The listing builds one solid part. Answer for the finished solid, in the listing's coordinates (mm). A direction names the side the tool comes from. Round coordinates to 2 decimals unless told otherwise and drop trailing zeros. Write each loop counter-clockwise with the first axis right and the second up, starting at its lowest first coordinate (ties: lowest second). Pieces come first, ordered by that corner, then holes. Notation, with made-up numbers: M 21,83 L 37,83 A17 ccw 37,116 Z; hole C -36.5,15 d2. An arc over 180 degrees is marked long. One line per item, written item: value. Start each with the question number.
(1) Consider probe 1 along Y at (x, z) = (2, 0.5); probe 2 along X at (y, z) = (1.2, 0); probe 3 along X at (y, z) = (-52, -0.75). Determine where each line is inside the solid, lowest interval first.
(2) For a pull along Z with two mould halves and no side action, classify faces 6 (the cylindrical face through (-4.21, 0.99, -0.38)), 7 (the cylindrical face through (4.285, -53.986, 4.199)), 8 (the flat face through (0, -53, 0)) as released by +Z, released by -Z, zero draft, split by the parting line, or undercut.
(3) Section C-C (x = 1.25) is taken. Determine the outline of the cut face in (y, z), plus the area to 3 significant figures.
(4) Given P1, Ø1.5, axis at x = 3, z = 2, coming from the +Y side; P2, Ø0.6, axis at y = 3, z = 0.5, coming from the -X side; P3, Ø4.5, axis at x = -2.5, z = 0, coming from the -Y side, each flat-ended and moving along its own axis, determine where each tip first touches the part or whether it passes through.
(5) For faces 1 (the flat face through (4, 3, -1)), 2 (the flat face through (-2, 0, -2)), 3 (the cylindrical face through (4.285, 2.986, 4.199)), 4 (the flat face through (4, -54, -1)), 5 (the flat face through (5, 4, 0)), determine the directions among +Z, -Z, +X, -X, +Y, -Y from which every point of the face is accessible in a straight line to the end or side of a thin tool.
(6) Section A-A (z = 0) is taken. Determine the outline of the cut face in (x, y).
(7) Section B-B (x = -2.5) is taken. Determine the outline of the cut face in (y, z), plus the area to 3 significant figures.
(8) Section D-D (z = 2.25) is taken. Determine the outline of the cut face in (x, y), plus the area to 3 significant figures.
```python
from build123d import *

# Parameters (mm, degrees)
SKETCH1_R           = 1.75
BOSS_EXTRUDE3_DEPTH = 2
BOSS_EXTRUDE4_DEPTH = 25.5
BOSS_EXTRUDE5_DEPTH = 4


with BuildPart() as part:
    # Sketch1 → Boss-Extrude3 (new body)
    # profile 1 of 3: a face of its own
    with BuildSketch(Plane(origin=(0, 0, 0), x_dir=(1, 0, 0), z_dir=(0, 1, 0))):
        with BuildLine():
            Line((0.004495957, 4.5), (-3.991008085, 4.5))
            ThreePointArc((-3.991008085, 4.5), (-7.240580672, 0), (-3.991008085, -4.5))
            Line((-3.991008085, -4.5), (0.004495957, -4.5))
            ThreePointArc((0.004495957, -4.5), (2.65, 0), (0.004495957, 4.5))
        make_face()
        with Locations(Location((-2.5, 0, 0), (0, 0, 270))):
            Circle(SKETCH1_R, mode=Mode.SUBTRACT)
    # profile 2 of 3: a face of its own
    with BuildSketch(Plane(origin=(0, 0, 0), x_dir=(1, 0, 0), z_dir=(0, 1, 0))):
        with BuildLine():
            Line((4, 4.5), (0.004495957, 4.5))
            ThreePointArc((0.004495957, 4.5), (2.65, 0), (0.004495957, -4.5))
            Line((0.004495957, -4.5), (4, -4.5))
            Line((4, -4.5), (5, -4.5))
            ThreePointArc((5, -4.5), (4.292893219, -4.207106781), (4, -3.5))
            Line((4, -3.5), (4, 4.5))
        make_face()
    # profile 3 of 3: a face of its own
    with BuildSketch(Plane(origin=(0, 0, 0), x_dir=(1, 0, 0), z_dir=(0, 1, 0))):
        with BuildLine():
            Line((5.019474666, 4.5), (4, 4.5))
            Line((4, 4.5), (4, -3.5))
            ThreePointArc((4, -3.5), (4.292893219, -4.207106781), (5, -4.5))
            Line((5, -4.5), (7, -4.5))
            Line((7, -4.5), (7, 4.5))
            Line((7, 4.5), (5.019474666, 4.5))
        make_face()
    extrude(amount=BOSS_EXTRUDE3_DEPTH)

    # Sketch1_3 → Boss-Extrude4 (add)
    with BuildSketch(Plane(origin=(0, 0, 0), x_dir=(1, 0, 0), z_dir=(0, 1, 0))):
        with BuildLine():
            ThreePointArc((0.004495957, 4.5), (2.65, 0), (0.004495957, -4.5))
            Line((0.004495957, -4.5), (7, -4.5))
            Line((7, -4.5), (7, 4.5))
            Line((7, 4.5), (0.004495957, 4.5))
        make_face()
    extrude(amount=-BOSS_EXTRUDE4_DEPTH)

    # Sketch1_5 → Boss-Extrude5 (add)
    with BuildSketch(Plane(origin=(0, 0, 0), x_dir=(1, 0, 0), z_dir=(0, 1, 0))):
        with BuildLine():
            Line((5.019474666, 4.5), (4, 4.5))
            Line((4, 4.5), (4, -3.5))
            ThreePointArc((4, -3.5), (4.292893219, -4.207106781), (5, -4.5))
            Line((5, -4.5), (7, -4.5))
            Line((7, -4.5), (7, 4.5))
            Line((7, 4.5), (5.019474666, 4.5))
        make_face()
    extrude(amount=BOSS_EXTRUDE5_DEPTH)

    # Mirror1: part across plane


with BuildPart() as part_1:
    add(part.part)
    add(part.part.mirror(Plane.ZX.offset(-25.5)))


solid = part_1.part
```
Recorded:
1. probe 1: y = -53 to -51, 0 to 2
1. probe 2: x = -7.24 to -4.25, -0.75 to 7
1. probe 3: x = -7.18 to -4.08, -0.92 to 7
2. face 6: undercut
2. face 7: released by +Z
2. face 8: zero draft
3. outline: M -53,-4.5 L 2,-4.5 L 2,4.5 L -53,4.5 Z; hole M -51,-3.53 L 0,-3.53 L 0,3.53 L -51,3.53 Z
3. area: 135 mm2
4. P1: stops at y = 2
4. P2: stops at x = 4
4. P3: stops at y = -53
5. face 1: +Z, -Z, -X, +Y
5. face 2: -X
5. face 3: +Z, -X, +Y
5. face 4: +Z, -Z, -X, -Y
5. face 5: +Z, -Z, +X, -X, +Y
6. outline: M -7.24,-53 L -4.25,-53 L -4.25,-51 L -7.24,-51 Z; M -7.24,0 L -4.25,0 L -4.25,2 L -7.24,2 Z; M -0.75,-53 L 4,-53 L 4,-55 L 7,-55 L 7,4 L 4,4 L 4,2 L -0.75,2 L -0.75,0 L 2.65,0 L 2.65,-51 L -0.75,-51 Z
7. outline: M -53,-4.5 L -51,-4.5 L -51,-1.75 L -53,-1.75 Z; M -53,1.75 L -51,1.75 L -51,4.5 L -53,4.5 Z; M 0,-4.5 L 2,-4.5 L 2,-1.75 L 0,-1.75 Z; M 0,1.75 L 2,1.75 L 2,4.5 L 0,4.5 Z
7. area: 22.0 mm2
8. outline: M -6.67,-53 L 4,-53 L 4,-55 L 7,-55 L 7,4 L 4,4 L 4,2 L -6.67,2 L -6.67,0 L 2.13,0 L 2.13,-51 L -6.67,-51 Z
8. area: 315 mm2
